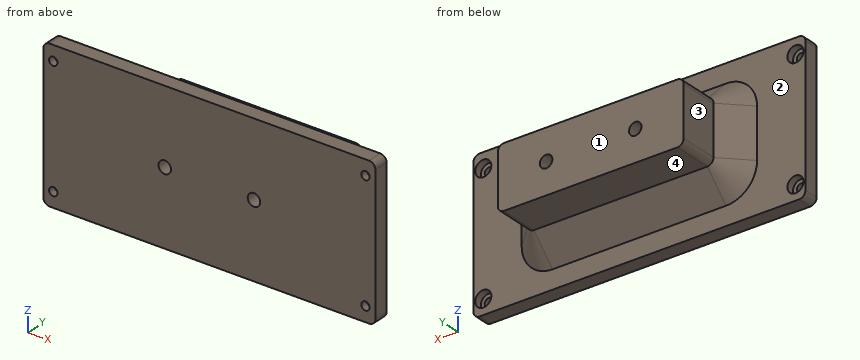
from build123d import *

# Parameters (mm, degrees)
SKETCH1_W                      = 134
SKETCH1_H                      = 60
BOSS_EXTRUDE1_DEPTH            = 6
CBORE_FOR_M3_SHCS1_D           = 3.4
CBORE_FOR_M3_SHCS1_DEPTH       = 17.38
CBORE_FOR_M3_SHCS1_CBORE_D     = 6.5
CBORE_FOR_M3_SHCS1_CBORE_DEPTH = 3
CBORE_FOR_M3_SHCS1_TIP         = 1.021463052
SKETCH4_W                      = 75
SKETCH4_H                      = 25
BOSS_EXTRUDE2_DEPTH            = 26
F_8_0_199_DIAMETER_HOLE1_D     = 5.0546
FILLET1_R                      = 2.5
FILLET2_R                      = 2.5
CHAMFER1_SIZE                  = 10


with BuildPart() as part:
    # Sketch1 → Boss-Extrude1 (new body)
    with BuildSketch(Plane(origin=(0, 0, 0), x_dir=(1, 0, 0), z_dir=(0, 1, 0))):
        Rectangle(SKETCH1_W, SKETCH1_H)
    extrude(amount=BOSS_EXTRUDE1_DEPTH)

    # CBORE for M3 SHCS1
    with Locations(Plane(origin=(0, 6, 0), x_dir=(1, 0, 0), z_dir=(0, 1, 0))):
        with Locations((-63, 24), (-63, -24), (63, -24), (63, 24)):
            CounterBoreHole(CBORE_FOR_M3_SHCS1_D / 2, CBORE_FOR_M3_SHCS1_CBORE_D / 2, CBORE_FOR_M3_SHCS1_CBORE_DEPTH, depth=CBORE_FOR_M3_SHCS1_DEPTH)
            with Locations((0, 0, -(CBORE_FOR_M3_SHCS1_DEPTH + CBORE_FOR_M3_SHCS1_TIP / 2))):  # 118° drill point
                Cone(0, CBORE_FOR_M3_SHCS1_D / 2, CBORE_FOR_M3_SHCS1_TIP, mode=Mode.SUBTRACT)

    # Sketch4 → Boss-Extrude2 (add)
    with BuildSketch(Plane(origin=(0, 6, 0), x_dir=(1, 0, 0), z_dir=(0, 1, 0))):
        Rectangle(SKETCH4_W, SKETCH4_H)
    extrude(amount=BOSS_EXTRUDE2_DEPTH)

    # #8 (0.199) Diameter Hole1 (through all)
    with Locations(Plane(origin=(0, 32, 0), x_dir=(1, 0, 0), z_dir=(0, 1, 0))):
        with Locations((-18, 0), (18, 0)):
            Hole(F_8_0_199_DIAMETER_HOLE1_D / 2)

    # Fillet1
    fillet1_edges = [part.edges().sort_by_distance(p)[0] for p in [
        (67, 3, 30),
        (-67, 3, 30),
        (-67, 3, -30),
        (67, 3, -30),
    ]]
    fillet(fillet1_edges, radius=FILLET1_R)

    # Fillet2
    fillet2_edges = [part.edges().sort_by_distance(p)[0] for p in [
        (37.5, 19, 12.5),
        (37.5, 19, -12.5),
        (-37.5, 19, -12.5),
        (-37.5, 19, 12.5),
    ]]
    fillet(fillet2_edges, radius=FILLET2_R)

    # Chamfer1
    chamfer1_edges = [part.edges().sort_by_distance(p)[0] for p in [
        (37.5, 6, 0),
        (0, 6, 12.5),
        (-37.5, 6, 0),
        (36.767766953, 6, -11.767766953),
        (36.767766953, 6, 11.767766953),
        (-36.767766953, 6, 11.767766953),
        (-36.767766953, 6, -11.767766953),
        (0, 6, -12.5),
    ]]
    chamfer(chamfer1_edges, length=CHAMFER1_SIZE)


solid = part.part
CAD build for the part. Positions are in the model's coordinates, mm. Face numbers are marked on the shaded views. A direction names the side the tool comes from. Round coordinates to 2 decimals unless told otherwise and drop trailing zeros. Loops run counter-clockwise (first coordinate to the right, second up) from the corner with the lowest first, then second, coordinate; pieces in that order, holes last. Notation, with made-up numbers: (-12.5, 59) - (22.5, 59) arc R13 ccw to (22.5, 78) - close; hole circle Ø9 at (18.25, 55.25). An arc over 180 degrees is marked (long way). Put each result on its own line as item: value.
1. Slice it at D-D on x = 63. List the corners of the cut face in (y, z).
Geometry check:
outline: (0, -30) - (6, -30) - (6, -27.25) - (3, -27.25) - (3, -25.7) - (0, -25.7) - close; (0, -22.3) - (3, -22.3) - (3, -20.75) - (6, -20.75) - (6, 20.75) - (3, 20.75) - (3, 22.3) - (0, 22.3) - close; (0, 25.7) - (3, 25.7) - (3, 27.25) - (6, 27.25) - (6, 30) - (0, 30) - close
2. Wall check: line 1 (X direction, y = 3.95, z = 24); line 2 (X direction, y = 1.95, z = 24); line 3 (Z direction, x = 18, y = 8). Give the ranges that are in metal, low to high.
Geometry check:
line 1: -67 to -66.25, -59.75 to 59.75, 66.25 to 67
line 2: -67 to -64.7, -61.3 to 61.3, 64.7 to 67
line 3: -20.5 to -2.53, 2.53 to 20.5
3. 3-axis set-ups, long thin cutter, end or side, ignore diameter. For the marked faces 1, 2, 3 and 4: which of +Z, -Z, +X, -X, +Y, -Y reach the whole face in a straight line?
Geometry check:
face 1: +Z, -Z, +X, -X, +Y
face 2: +Y
face 3: +Z, -Z, -X, +Y
face 4: -Z, +X, -X, +Y
4. Slice it at A-A on z = -24. List the corners of the cut face in (x, y), and give its area (3 significant figures).
Geometry check:
outline: (-67, 0) - (-64.7, 0) - (-64.7, 3) - (-66.25, 3) - (-66.25, 6) - (-67, 6) - close; (-61.3, 0) - (61.3, 0) - (61.3, 3) - (59.75, 3) - (59.75, 6) - (-59.75, 6) - (-59.75, 3) - (-61.3, 3) - close; (64.7, 0) - (67, 0) - (67, 6) - (66.25, 6) - (66.25, 3) - (64.7, 3) - close
area: 745 mm²
5. Pin check, flat tips, straight feed: P1, Ø3, axis at y = 7, z = -12.5, coming from the +X side; P2, Ø5, axis at x = -63, z = -25, coming from the +Y side; P3, Ø5, axis at x = 12, y = 28, coming from the +Z side; P4, Ø1, axis at y = 28, z = -12.5, coming from the +X side. Stop position of each tip, or through.
Geometry check:
P1: x = 67
P2: y = 6
P3: z = 12.5
P4: x = 36.5
6. Slice it at C-C on y = 8. List the corners of the cut face in (x, z).
Geometry check:
outline: (-45.5, -10) arc R10.5 ccw to (-35, -20.5) - (35, -20.5) arc R10.5 ccw to (45.5, -10) - (45.5, 10) arc R10.5 ccw to (35, 20.5) - (-35, 20.5) arc R10.5 ccw to (-45.5, 10) - close; hole circle Ø5.05 at (-18, 0); hole circle Ø5.05 at (18, 0)
7. Slice it at B-B on x = -18. List the corners of the cut face in (y, z), and give its area (3 significant figures).
Geometry check:
outline: (0, -30) - (6, -30) - (6, -22.5) - (16, -12.5) - (32, -12.5) - (32, -2.53) - (0, -2.53) - close; (0, 2.53) - (32, 2.53) - (32, 12.5) - (16, 12.5) - (6, 22.5) - (6, 30) - (0, 30) - close
area: 948 mm²
